Geometry: final body of the model. Coordinates: model frame, mm. Face numbers are marked on the shaded views. A direction names the side the tool comes from. Give positions to 0.01 mm unless a question says otherwise; leave off trailing zeros. Order: outer loops, then holes, each group sorted by start corner. A loop starts at its lowest first (then second) coordinate and runs counter-clockwise, first axis right, second up. Notation, with made-up numbers: (-7.5, 85.25) -> (17.5, 85.25) arc R15 cw to (17.5, 109.25) -> close; hole circle Ø1 at (87, 33.5). An arc over 180 degrees is marked (long way). Answer in a Markdown table with one row per item. Add a question column.
Q1. Contact query for flat-ended pins moving along their axis: P1, Ø10, axis at x = 155, y = 62, coming from the +Z side; P2, Ø2.5, axis at x = -80, y = 15, coming from the -Z side; P3, Ø3, axis at x = 46.5, y = 38, coming from the +Z side; P4, Ø3, axis at x = 233.25, y = -30, coming from the -Z side. Output: stop coordinate, or through.
Q2. Cut plane C-C on z = 0.9. Count the separate pieces of the cut face and the enclosed holes in it, and give its area (3 significant figures).
Q3. Cut plane B-B on y = 71. Return the cut outline in (x, z), and give its area (3 significant figures).
Q4. Cut plane A-A on y = 45. Return the cut outline in (x, z).
Q5. Line query: line 1 along Y through (x, z) = (303, 2.9); line 2 along Y through (x, z) = (83, 0.8); line 3 along X through (y, z) = (38, 0.4). Output: solid intervals per line, ascending. Write a range as from..to.
Q6. Set-up query: the marked faces 1 and 2. Return all of +Z, -Z, +X, -X, +Y, -Y with unobstructed straight access to the full face (end or side cutting, diameter ignored); none if empty.
from build123d import *

# Parameters (mm, degrees)
EXTRUDE_1_DEPTH             = 3
SKETCH_2_W                  = 190
SKETCH_2_H                  = 5
SKETCH_2_H_2                = 20
CUT_EXTRUDE_1_DEPTH         = 4
SKETCH_3_W                  = 200
SKETCH_3_H                  = 70
CUT_EXTRUDE_2_DEPTH         = 1
EXTRUDE_2_DEPTH             = 3
CHAMFER_1_SIZE              = 15
HOLE_WIZARD_M41_D           = 3.3
HOLE_WIZARD_M41_DEPTH       = 11.5
HOLE_WIZARD_M41_CSINK_D     = 4.05
HOLE_WIZARD_M41_CSINK_ANGLE = 120
HOLE_WIZARD_M41_TIP         = 0.991420021
HOLE_WIZARD_M31_D           = 2.5
HOLE_WIZARD_M31_DEPTH       = 8.5
HOLE_WIZARD_M31_CSINK_D     = 3.05
HOLE_WIZARD_M31_CSINK_ANGLE = 120
HOLE_WIZARD_M31_TIP         = 0.751075774
HOLE_WIZARD_M32_D           = 2.5
HOLE_WIZARD_M32_DEPTH       = 8.5
HOLE_WIZARD_M32_CSINK_D     = 3.05
HOLE_WIZARD_M32_CSINK_ANGLE = 120
HOLE_WIZARD_M32_TIP         = 0.751075774
HOLE_WIZARD_M42_D           = 4.5
HOLE_WIZARD_M42_DEPTH       = 5
HOLE_WIZARD_M42_TIP         = 1.351936393


with BuildPart() as part:
    # Эскиз1 → Бобышка-Вытянуть1 (new body)
    with BuildSketch(Plane.XY):
        Polygon((259, 50), (298, 50), (298, 0), (0, 0), (0, 50), (39, 50), (39, 90), (259, 90), align=None)
    extrude(amount=EXTRUDE_1_DEPTH)

    # Эскиз2 → Вырез-Вытянуть1 (cut)
    with BuildSketch(Plane.XY.offset(3)):
        with Locations((149, 80.5)):
            Rectangle(SKETCH_2_W, SKETCH_2_H)
        with Locations((149, 50)):
            Rectangle(SKETCH_2_W, SKETCH_2_H_2)
    extrude(amount=-CUT_EXTRUDE_1_DEPTH, mode=Mode.SUBTRACT)

    # Эскиз3 → Вырез-Вытянуть2 (cut)
    with BuildSketch(Plane.XY.offset(3)):
        with Locations((149, 55)):
            Rectangle(SKETCH_3_W, SKETCH_3_H)
    extrude(amount=-CUT_EXTRUDE_2_DEPTH, mode=Mode.SUBTRACT)

    # Эскиз4 → Бобышка-Вытянуть2 (add)
    with BuildSketch(Plane.XY.offset(3)):
        Polygon((0, 50), (-100, 50), (-100, 0), (-60, 0), (-60, -38), (318, -38), (318, 0), (358, 0), (358, 50), (298, 50), (298, 0), (0, 0), align=None)
    extrude(amount=-EXTRUDE_2_DEPTH)

    # Фаска1
    chamfer_1_edges = [part.edges().sort_by_distance(p)[0] for p in [
        (39, 50, 1.5),
        (259, 50, 1.5),
    ]]
    chamfer(chamfer_1_edges, length=CHAMFER_1_SIZE)

    # Отверстие обработанное метчиком M41
    with Locations(Plane.XY.offset(3)):
        with Locations((-46, -30), (-26, -30), (-46, -10), (-26, -10), (284, -10), (304, -10), (304, -30), (284, -30)):
            CounterSinkHole(HOLE_WIZARD_M41_D / 2, HOLE_WIZARD_M41_CSINK_D / 2, depth=HOLE_WIZARD_M41_DEPTH, counter_sink_angle=HOLE_WIZARD_M41_CSINK_ANGLE)
            with Locations((0, 0, -(HOLE_WIZARD_M41_DEPTH + HOLE_WIZARD_M41_TIP / 2))):  # 118° drill point
                Cone(0, HOLE_WIZARD_M41_D / 2, HOLE_WIZARD_M41_TIP, mode=Mode.SUBTRACT)

    # Отверстие обработанное метчиком M31
    with Locations(Plane(origin=(0, 0, 0), x_dir=(-1, 0, 0), z_dir=(0, 0, -1))):
        with Locations((-268, -30), (-233.25, -30), (-198.5, -30), (-163.75, -30), (-129, -30), (-94.25, -30), (-59.5, -30), (-24.75, -30), (10, -30)):
            CounterSinkHole(HOLE_WIZARD_M31_D / 2, HOLE_WIZARD_M31_CSINK_D / 2, depth=HOLE_WIZARD_M31_DEPTH, counter_sink_angle=HOLE_WIZARD_M31_CSINK_ANGLE)
            with Locations((0, 0, -(HOLE_WIZARD_M31_DEPTH + HOLE_WIZARD_M31_TIP / 2))):  # 118° drill point
                Cone(0, HOLE_WIZARD_M31_D / 2, HOLE_WIZARD_M31_TIP, mode=Mode.SUBTRACT)

    # Отверстие обработанное метчиком M32
    with Locations(Plane.XY.offset(3)):
        with Locations((251.5, 82), (46.5, 82), (251.5, 60), (46.5, 60), (251.5, 38), (46.5, 38), (251.5, 16), (46.5, 16)):
            CounterSinkHole(HOLE_WIZARD_M32_D / 2, HOLE_WIZARD_M32_CSINK_D / 2, depth=HOLE_WIZARD_M32_DEPTH, counter_sink_angle=HOLE_WIZARD_M32_CSINK_ANGLE)
            with Locations((0, 0, -(HOLE_WIZARD_M32_DEPTH + HOLE_WIZARD_M32_TIP / 2))):  # 118° drill point
                Cone(0, HOLE_WIZARD_M32_D / 2, HOLE_WIZARD_M32_TIP, mode=Mode.SUBTRACT)

    # Отверстие с зазором M42
    with Locations(Plane.XY.offset(3)):
        with Locations((338, 15), (285.75, 15), (233.5, 15), (181.25, 15), (129, 15), (76.75, 15), (24.5, 15), (-27.75, 15), (-80, 15)):
            Hole(HOLE_WIZARD_M42_D / 2, depth=HOLE_WIZARD_M42_DEPTH)
            with Locations((0, 0, -(HOLE_WIZARD_M42_DEPTH + HOLE_WIZARD_M42_TIP / 2))):  # 118° drill point
                Cone(0, HOLE_WIZARD_M42_D / 2, HOLE_WIZARD_M42_TIP, mode=Mode.SUBTRACT)


solid = part.part
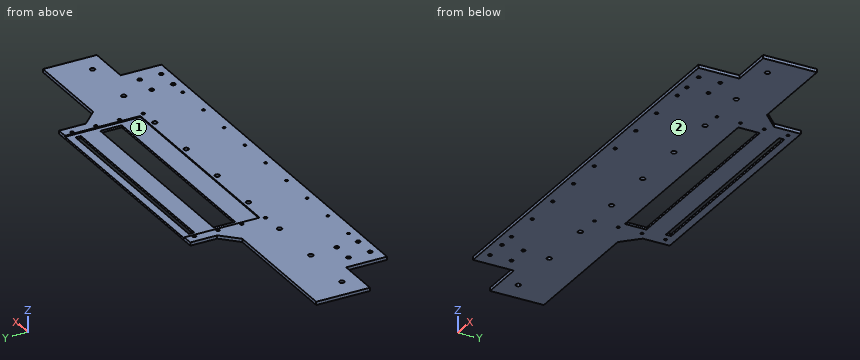
Completed:
| question | item | result |
|---|---|---|
| 1 | P1 | stops at z = 2 |
| 1 | P2 | passes through |
| 1 | P3 | stops at z = 2.99 |
| 1 | P4 | stops at z = 0.01 |
| 2 | separate pieces | 1 |
| 2 | enclosed holes | 36 |
| 2 | area | 41,200 mm² |
| 3 | outline | (39, 0) -> (259, 0) -> (259, 3) -> (249, 3) -> (249, 2) -> (49, 2) -> (49, 3) -> (39, 3) -> close |
| 3 | area | 460 mm² |
| 4 | outline | (-100, 0) -> (54, 0) -> (54, 2) -> (49, 2) -> (49, 3) -> (-100, 3) -> close; (244, 0) -> (358, 0) -> (358, 3) -> (249, 3) -> (249, 2) -> (244, 2) -> close |
| 5 | line 1 | y = -38..-31.56, -28.44..-11.56, -8.44..50 |
| 5 | line 2 | y = -38..40, 60..78, 83..90 |
| 5 | line 3 | x = -100..45.25, 47.75..250.25, 252.75..358 |
| 6 | face 1 | +Z, +Y |
| 6 | face 2 | -Z, +X, -X, +Y, -Y |
